```python
from build123d import *

# Parameters (mm, degrees)
F1_DEPTH = 6.35
F2_R     = 1.27
F3_R     = 0.254
F5_DEPTH = 2.5236418215


with BuildPart() as f1:
    # F0 (on Right) → F1 (new body, symmetric)
    with BuildSketch(Plane.YZ):
        with BuildLine():
            Line((-20.3536781971, 19.8174831357), (9.2510120329, 16.4412551424))
            Line((9.2510120329, 16.4412551424), (9.2510120329, 18.9812551424))
            Line((9.2510120329, 18.9812551424), (-21.8487802355, 22.5279900829))
            ThreePointArc((-21.8487802355, 22.5279900829), (-22.7318674452, 22.2475119605), (-23.1106011462, 21.4018927905))
            Line((-23.1106011462, 21.4018927905), (-23.1106011462, -18.4179837987))
            Line((-23.1106011462, -18.4179837987), (-20.5706011462, -18.4179837987))
            Line((-20.5706011462, -18.4179837987), (-20.5706011462, 19.6238927905))
            ThreePointArc((-20.5706011462, 19.6238927905), (-20.5054920403, 19.7692654045), (-20.3536781971, 19.8174831357))
        make_face()
    extrude(amount=F1_DEPTH, both=True)

    # F2
    f2_edges = [f1.edges().sort_by_distance(p)[0] for p in [
        (6.35, 9.251012, 17.711255),
        (-6.35, 9.251012, 17.711255),
        (-6.35, -21.840601, -18.417984),
        (6.35, -21.840601, -18.417984),
    ]]
    fillet(f2_edges, radius=F2_R)

    # F3
    f3_edges = [f1.edges().sort_by_distance(p)[0] for p in [
        (6.35, -23.110601, 2.126954),
        (6.35, -20.570601, 1.237954),
    ]]
    fillet(f3_edges, radius=F3_R)

    # F4 (on face) → F5 (cut, through all)
    with BuildSketch(Plane(origin=(0, 2.2556734095, 19.779029343), x_dir=(1, 0, 0), z_dir=(0, 0.1133092186, 0.9935597722))):
        with BuildLine():
            Line((2.3688334775, -2.1236329222), (-2.2031665225, -2.1236329222))
            ThreePointArc((-2.2031665225, -2.1236329222), (-2.382771645, -2.1980277998), (-2.4571665225, -2.3776329222))
            Line((-2.4571665225, -2.3776329222), (-2.4571665225, -15.0776329222))
            ThreePointArc((-2.4571665225, -15.0776329222), (-2.382771645, -15.2572380446), (-2.2031665225, -15.3316329222))
            Line((-2.2031665225, -15.3316329222), (2.3688334775, -15.3316329222))
            ThreePointArc((2.3688334775, -15.3316329222), (2.5484385999, -15.2572380446), (2.6228334775, -15.0776329222))
            Line((2.6228334775, -15.0776329222), (2.6228334775, -2.3776329222))
            ThreePointArc((2.6228334775, -2.3776329222), (2.5484385999, -2.1980277998), (2.3688334775, -2.1236329222))
        make_face()
    extrude(amount=-F5_DEPTH, mode=Mode.SUBTRACT)


solid = f1.part
```
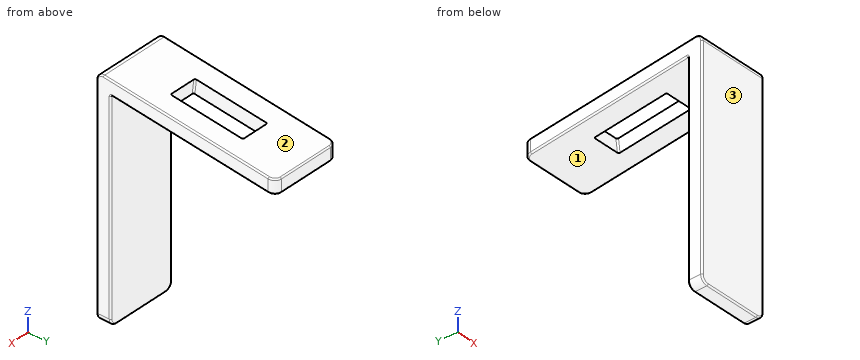
For this review, take the finished solid that the model builds, in its own axes (mm). Face numbers are marked on the shaded views. Coordinates: 2 decimals unless noted, no trailing zeros. Write each loop counter-clockwise with the first axis right and the second up, starting at its lowest first coordinate (ties: lowest second). Pieces come first, ordered by that corner, then holes. Notation, with made-up numbers: (80, 52.5) - (105, 52.5) arc R12 ccw to (105, 74.5) - close; hole circle Ø5 at (81.25, -35). An arc over 180 degrees is marked (long way). Answer in a Markdown table with one row per item. Add a question column.
Q1. We need section C-C, the plane x = -4.5. State the section outline as (y, z) points, and give its area (3 significant figures).
Q2. We need section B-B, the plane z = 4. State the section outline as (x, y) points.
Q3. For probe 1 along Y at (x, z) = (2, -14); probe 2 along Z at (x, y) = (-0.75, 7.5); probe 3 along Z at (x, y) = (-4.75, 2), list the stretches that pass through material, from the lowest coordinate up.
Q4. For P1, Ø5, axis at x = 4, y = 6, coming from the -Z side; P2, Ø6, axis at x = 2, y = -6, coming from the -Z side; P3, Ø4, axis at x = -3, y = -19, coming from the +Z side, all flat-tipped, find the tip position at first contact; note any pin that passes through.
Q5. Draft analysis for pull direction Y (two halves, no side actions). For the marked faces 1, 2 and 3, state which applies: +Y half, -Y half, draft (parallel to the pull), parting line (faces both ways), or undercut.
Q6. We need section A-A, the plane x = -0.5. State the section outline as (y, z) points.
Answer list:
| question | item | result |
|---|---|---|
| 1 | outline | (-23.11, -18.16) arc R0.25 ccw to (-22.86, -18.42) - (-20.82, -18.42) arc R0.25 ccw to (-20.57, -18.16) - (-20.57, 19.62) arc R0.19 cw to (-20.35, 19.82) - (8.97, 16.47) arc R0.25 ccw to (9.25, 16.73) - (9.25, 18.75) arc R0.25 ccw to (9.03, 19.01) - (-21.85, 22.53) arc R1.13 ccw to (-23.11, 21.4) - close |
| 1 | area | 179 mm2 |
| 2 | outline | (-6.35, -22.86) arc R0.25 ccw to (-6.1, -23.11) - (6.1, -23.11) arc R0.25 ccw to (6.35, -22.86) - (6.35, -20.82) arc R0.25 ccw to (6.1, -20.57) - (-6.1, -20.57) arc R0.25 ccw to (-6.35, -20.82) - close |
| 3 | probe 1 | y = -23.11 to -20.57 |
| 3 | probe 2 | z = 16.64 to 19.18 |
| 3 | probe 3 | z = 17.27 to 19.81 |
| 4 | P1 | stops at z = 16.53 |
| 4 | P2 | stops at z = 17.85 |
| 4 | P3 | stops at z = 22.43 |
| 5 | face 1 | undercut |
| 5 | face 2 | +Y half |
| 5 | face 3 | -Y half |
| 6 | outline | (-23.11, -18.16) arc R0.25 ccw to (-22.86, -18.42) - (-20.82, -18.42) arc R0.25 ccw to (-20.57, -18.16) - (-20.57, 19.62) arc R0.19 cw to (-20.35, 19.82) - (-13.26, 19.01) - (-12.98, 21.52) - (-21.85, 22.53) arc R1.13 ccw to (-23.11, 21.4) - close; (-0.14, 17.51) - (8.97, 16.47) arc R0.25 ccw to (9.25, 16.73) - (9.25, 18.75) arc R0.25 ccw to (9.03, 19.01) - (0.15, 20.02) - close |
